Print and shaded views of the part. All mm, measured from the part's lowest x, y and z. Coordinates: 2 decimals unless noted, no trailing zeros. Order: outer loops, then holes, each group sorted by start corner. A loop starts at its lowest first (then second) coordinate and runs counter-clockwise, first axis right, second up.
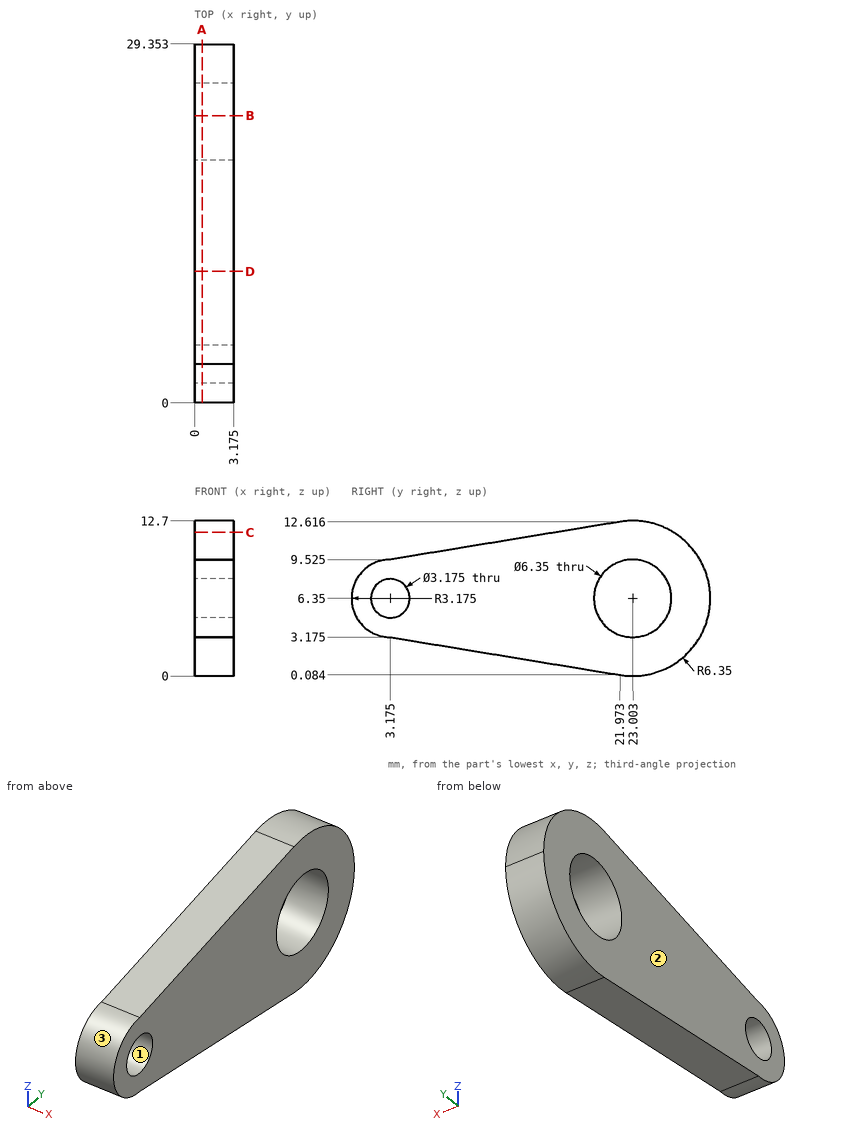
Q1. Cut at C-C, the plane z = 11.75. List the corners of the cut face in (x, y) (1 decimal), plus the area to 3 significant figures.
Established:
outline: (0, 16.7) - (3.2, 16.7) - (3.2, 26.3) - (0, 26.3) - close
area: 30.6 mm2
Q2. Drop flat-ended pins along their axis: P1, Ø5, axis at y = 3.175, z = 6.35, coming from the +X side (3 decimals); P2, Ø1.5, axis at x = 2.5, z = 11, coming from the +Y side (1 decimal). Give the stop position or say it passes through.
Established:
P1: stops at x = 3.175
P2: stops at y = 28
Q3. Cut at D-D, the plane y = 10.75. List the corners of the cut face in (x, z) (1 decimal).
Established:
outline: (0, 1.9) - (3.2, 1.9) - (3.2, 10.8) - (0, 10.8) - close
Q4. Probe line 1 (Y direction, x = 2.35, z = 7.25); line 2 (Y direction, x = 2.15, z = 7) (1 decimal); line 3 (Z direction, x = 2.55, y = 4) (1 decimal). List the from-to ranges inside material, lowest first.
Established:
line 1: y = 0.13 to 1.87, 4.48 to 19.96, 26.05 to 29.29
line 2: y = 0.1 to 1.7, 4.6 to 19.9, 26.1 to 29.3
line 3: z = 3 to 5, 7.7 to 9.7
Q5. Mould opens along Y. For the marked faces 1, 2 and 3 say: pulls with the +Y half, pulls with the -Y half, needs draft (parallel to the pull), parting line crosses it, or undercut.
Established:
face 1: undercut
face 2: needs draft
face 3: pulls with the -Y half
Q6. Cut at A-A, the plane x = 0.6. Count the separate pieces of the cut face and the enclosed holes in it, plus the area to 3 significant figures.
Established:
separate pieces: 1
enclosed holes: 2
area: 230 mm2
Q7. Cut at B-B, the plane y = 23.5. List the corners of the cut face in (x, z) (1 decimal).
Established:
outline: (0, 0) - (3.2, 0) - (3.2, 3.2) - (0, 3.2) - close; (0, 9.5) - (3.2, 9.5) - (3.2, 12.7) - (0, 12.7) - close
